Answer from the drawing. Dimensions are ordinates in mm from the lowest x, y and z of the part. Coordinates: 2 decimals unless noted, no trailing zeros. Order: outer loops, then holes, each group sorted by start corner. A loop starts at its lowest first (then second) coordinate and runs counter-clockwise, first axis right, second up. Notation, with made-up numbers: (17, 43) -> (45, 43) arc R12 ccw to (45, 56) -> close; hole circle Ø3 at (-14.75, 71.25). An arc over 180 degrees is marked (long way). Use CSV: the item, a comma, the result in double quotes.
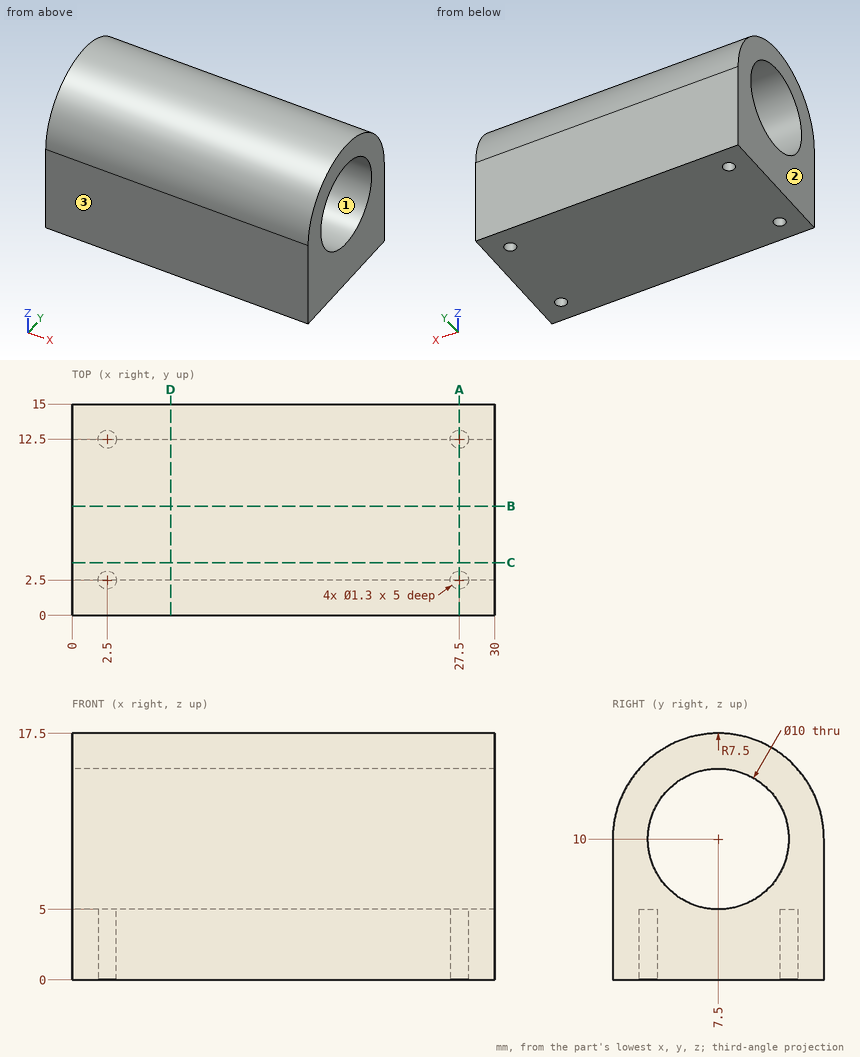
Item 1: Find section B-B, the plane y = 7.75. Give the vertices of the cut face in (x, z).
Return value:
outline,"(0, 0) -> (30, 0) -> (30, 5.01) -> (0, 5.01) -> close; (0, 14.99) -> (30, 14.99) -> (30, 17.5) -> (0, 17.5) -> close"
Item 2: Find section D-D, the plane x = 7. Give the vertices of the cut face in (y, z).
Return value:
outline,"(0, 0) -> (15, 0) -> (15, 10) arc R7.5 ccw to (0, 10) -> close; hole circle Ø10 at (7.5, 10)"
Item 3: Find section A-A, the plane x = 27.5. Give the vertices of the cut face in (y, z), then the cut area to 3 significant figures.
Return value:
outline,"(0, 0) -> (1.85, 0) -> (1.85, 5) -> (3.15, 5) -> (3.15, 0) -> (11.85, 0) -> (11.85, 5) -> (13.15, 5) -> (13.15, 0) -> (15, 0) -> (15, 10) arc R7.5 ccw to (0, 10) -> close; hole circle Ø10 at (7.5, 10)"
area,"147 mm^2"
Item 4: Straight lines are drawn through the part: line 1 along Y through (x, z) = (2.5, 3.25); line 2 along X through (y, z) = (12.5, 2.85); line 3 along Z through (x, y) = (15.25, 7.25). For each, find the intervals that lie inside material, in ascending order.
Return value:
line 1,"y = 0 to 1.85, 3.15 to 11.85, 13.15 to 15"
line 2,"x = 0 to 1.85, 3.15 to 26.85, 28.15 to 30"
line 3,"z = 0 to 5.01, 14.99 to 17.5"
Item 5: Each of these flat-tipped pins is pushed along its axis until it touches: P1, Ø1, axis at x = 2.5, y = 12.5, coming from the -Z side; P2, Ø1, axis at x = 2.5, y = 2.5, coming from the +Z side; P3, Ø1.7, axis at x = 27.5, y = 12.5, coming from the +Z side. Where does it stop, or does it pass through?
Return value:
P1,"stops at z = 5"
P2,"stops at z = 16"
P3,"stops at z = 16.25"
Item 6: Find section C-C, the plane y = 3.75. Give the vertices of the cut face in (x, z), then the cut area to 3 significant figures.
Return value:
outline,"(0, 0) -> (30, 0) -> (30, 6.69) -> (0, 6.69) -> close; (0, 13.31) -> (30, 13.31) -> (30, 16.5) -> (0, 16.5) -> close"
area,"296 mm^2"
Item 7: The mould has two halves that part along Y. Classify the marked faces 1, 2 and 3: +Y half, -Y half, draft (parallel to the pull), parting line (faces both ways), or undercut.
Return value:
face 1,"undercut"
face 2,"draft"
face 3,"-Y half"
